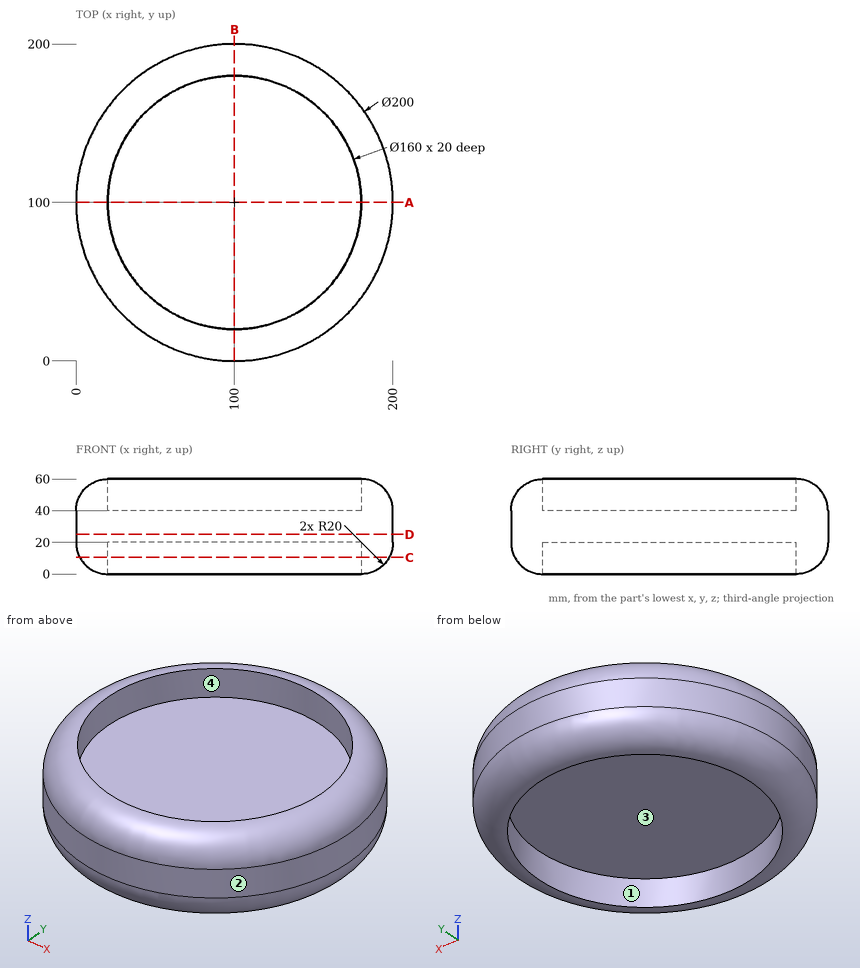
Print and shaded views of the part. All mm, measured from the part's lowest x, y and z. A direction names the side the tool comes from. Coordinates: 2 decimals unless noted, no trailing zeros. Loops run counter-clockwise (first coordinate to the right, second up) from the corner with the lowest first, then second, coordinate; pieces in that order, holes last. Notation, with made-up numbers: (-11.5, 33) - (-2.5, 33) arc R32 cw to (-2.5, 61) - close; hole circle Ø1 at (19, 87.5). An arc over 180 degrees is marked (long way). Use one line per item in the form item = value. Start each with the question number.
1) Flat gauge pins, fed straight in: pin 1 (12 mm diameter, centred on x = 139.5, z = 16.5, fed in from +Y); pin 2 (1.5 mm diameter, centred on x = 40, z = 38.5, fed in from +Y); pin 3 (5 mm diameter, centred on x = 108.5, y = 46, fed in from -Z). Where does each tip first touch, or does it go through?
2) Two-plate mould, pull along X, no slides. Class the marked faces 1 and 2: +X half, -X half, draft (parallel to the pull), parting line (faces both ways), or undercut.
3) Band-saw the part on C-C (z = 10.5). Give the cut face in (x, y), and give its area (3 significant figures).
4) Drill centre lines: L1, parallel to Y at x = 100, z = 23; L2, parallel to Z at x = 142.5, y = 117; L3, parallel to Y at x = 44, z = 52. Where is each one in solid material? Low to high. Write a range as from..to.
5) Band-saw the part on D-D (z = 25). Give the cut face in (x, y), and give its area (3 significant figures).
6) Band-saw the part on A-A (y = 100). Give the cut face in (x, z).
7) Tool access for the marked faces 3 and 4: list every direction of +Z, -Z, +X, -X, +Y, -Y with a clear straight run to the whole face (end or side of a thin tool).
Check values:
q1.pin_1 = 194.05
q1.pin_2 = 180.56
q1.pin_3 = 20
q2.face_1 = undercut
q2.face_2 = parting line
q3.outline = circle Ø195.2 at (100, 100); hole circle Ø160 at (100, 100)
q3.area = 9,820 mm2
q4.L1 = 0..200
q4.L2 = 20..40
q4.L3 = 22.03..42.87, 157.13..177.97
q5.outline = circle Ø200 at (100, 100)
q5.area = 31,400 mm2
q6.outline = (0, 20) arc R20 ccw to (20, 0) - (20, 20) - (180, 20) - (180, 0) arc R20 ccw to (200, 20) - (200, 40) arc R20 ccw to (180, 60) - (180, 40) - (20, 40) - (20, 60) arc R20 ccw to (0, 40) - close
q7.face_3 = -Z
q7.face_4 = +Z
